Design review of the part built by this model. Coordinates are the model's own, in mm. Give positions to 0.01 mm unless a question says otherwise; leave off trailing zeros. Loops run counter-clockwise (first coordinate to the right, second up) from the corner with the lowest first, then second, coordinate; pieces in that order, holes last.
from build123d import *

# Parameters (mm, degrees)
SKETCH_1_W          = 250
SKETCH_1_H          = 250
EXTRUDE_1_DEPTH     = 3
SKETCH_3_W          = 132
SKETCH_3_H          = 200
CUT_EXTRUDE_1_DEPTH = 10
SKETCH_4_R          = 1.25
CUT_EXTRUDE_2_DEPTH = 10


with BuildPart() as part:
    # Эскиз1 → Бобышка-Вытянуть1 (new body)
    with BuildSketch(Plane(origin=(0, 0, 0), x_dir=(1, 0, 0), z_dir=(0, 1, 0))):
        Rectangle(SKETCH_1_W, SKETCH_1_H)
    extrude(amount=EXTRUDE_1_DEPTH)

    # Эскиз3 → Вырез-Вытянуть1 (cut)
    with BuildSketch(Plane.XZ):
        with Locations((34, 0)):
            Rectangle(SKETCH_3_W, SKETCH_3_H)
    extrude(amount=-CUT_EXTRUDE_1_DEPTH, mode=Mode.SUBTRACT)

    # Эскиз4 → Вырез-Вытянуть2 (cut)
    with BuildSketch(Plane.XZ):
        with Locations(Location((-121, 121, 0), (0, 0, 270))):
            Circle(SKETCH_4_R)
        with Locations(Location((121, 121, 0), (0, 0, 270))):
            Circle(SKETCH_4_R)
        with Locations(Location((121, -121, 0), (0, 0, 270))):
            Circle(SKETCH_4_R)
        with Locations(Location((-121, -121, 0), (0, 0, 270))):
            Circle(SKETCH_4_R)
    extrude(amount=-CUT_EXTRUDE_2_DEPTH, mode=Mode.SUBTRACT)


solid = part.part
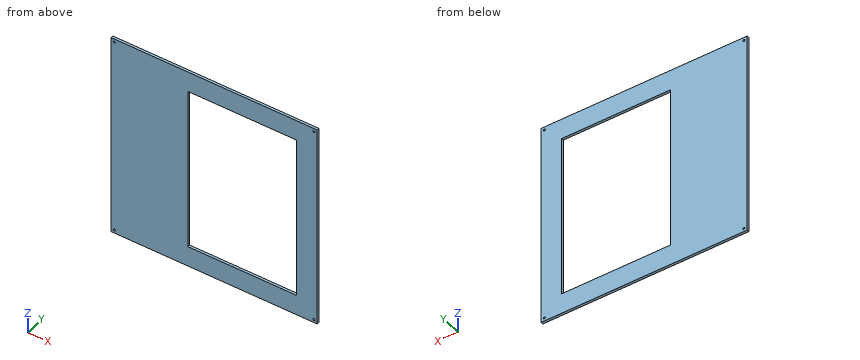
Q1. Take a section at C-C (y = 0.7). Give the boundary of the cut face in (x, z).
Results:
outline: (-125, -125) - (125, -125) - (125, 125) - (-125, 125) - close; hole circle Ø2.5 at (-121, -121); hole circle Ø2.5 at (-121, 121); hole (-32, -100) - (100, -100) - (100, 100) - (-32, 100) - close; hole circle Ø2.5 at (121, -121); hole circle Ø2.5 at (121, 121)
Q2. Wall thickness on line 1 (Z direction, x = -121, y = 1.2); line 2 (X direction, y = 2.75, z = -54.5): over which ranges is each line inside the solid? List them lowest first.
Results:
line 1: z = -125 to -122.25, -119.75 to 119.75, 122.25 to 125
line 2: x = -125 to -32, 100 to 125
Q3. Insertion check: pin 1 (1.5 mm diameter, centred on x = -121, z = -121, fed in from +Y) (3 decimals). The pin has a flat end and moves straight along its axis. Give the tip position at first contact, or say it passes through.
Results:
pin 1: passes through
Q4. Take a section at B-B (x = 7.5). Give the boundary of the cut face in (y, z).
Results:
outline: (0, -125) - (3, -125) - (3, -100) - (0, -100) - close; (0, 100) - (3, 100) - (3, 125) - (0, 125) - close
Q5. Take a section at A-A (z = -84). Give the boundary of the cut face in (x, y).
Results:
outline: (-125, 0) - (-32, 0) - (-32, 3) - (-125, 3) - close; (100, 0) - (125, 0) - (125, 3) - (100, 3) - close
